Verification items for the finished model (mm, model axes). Face numbers are marked on the shaded views. Round coordinates to 2 decimals unless told otherwise and drop trailing zeros. Loops run counter-clockwise (first coordinate to the right, second up) from the corner with the lowest first, then second, coordinate; pieces in that order, holes last. Notation, with made-up numbers: M 19.25,9 L 50.25,9 A15 ccw 50.25,35 Z; hole C 2.25,23.25 d4. An arc over 180 degrees is marked long. One line per item, written item: value.
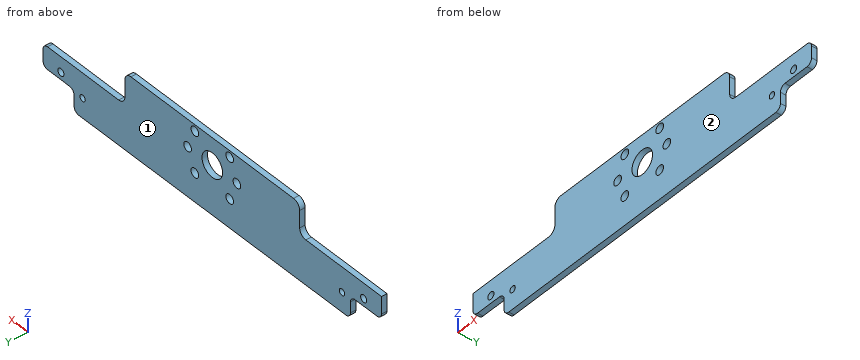
from build123d import *

# Parameters (mm, degrees)
SKETCH_2_R      = 2.5
SKETCH_2_R_2    = 2.499999999
SKETCH_2_R_3    = 6.682030953
SKETCH_2_R_4    = 2
SKETCH_2_R_5    = 1.75
EXTRUDE_1_DEPTH = 3
FILLET_1_R      = 4
FILLET_2_R      = 3


with BuildPart() as part:
    # 草图2 → 凸台-拉伸1 (new body)
    with BuildSketch(Plane(origin=(0, 0, 0), x_dir=(1, 0, 0), z_dir=(0, 1, 0))):
        Polygon((56.805521657, -9.129480985), (110, -9.129480985), (110, 3.251695679), (89.78, 3.370519015), (89.78, 15.370519015), (-89.78, 15.370519015), (-89.78, 3.370519015), (-110, 3.370519015), (-110, -9.129480985), (-56.805521657, -9.129480985), (-56.805521657, -26.629480985), (56.805521657, -26.629480985), align=None)
        with Locations((-16.000000001, -11.748304322)):
            Circle(SKETCH_2_R, mode=Mode.SUBTRACT)
        with Locations((-11.313708499, -23.062012821)):
            Circle(SKETCH_2_R_2, mode=Mode.SUBTRACT)
        with Locations((-11.3137085, -0.434595823)):
            Circle(SKETCH_2_R, mode=Mode.SUBTRACT)
        with Locations((0, -11.748304321)):
            Circle(SKETCH_2_R_3, mode=Mode.SUBTRACT)
        with Locations((11.313708498, -0.434595822)):
            Circle(SKETCH_2_R, mode=Mode.SUBTRACT)
        with Locations((16, -11.748304321)):
            Circle(SKETCH_2_R, mode=Mode.SUBTRACT)
        with Locations((11.313708499, -23.062012821)):
            Circle(SKETCH_2_R_2, mode=Mode.SUBTRACT)
        with Locations((98.383175919, -0.748304322)):
            Circle(SKETCH_2_R_4, mode=Mode.SUBTRACT)
        with Locations((84.28, 4.561107346)):
            Circle(SKETCH_2_R_5, mode=Mode.SUBTRACT)
        with Locations((-84.280000001, 4.561107346)):
            Circle(SKETCH_2_R_5, mode=Mode.SUBTRACT)
        with Locations((-98.38317592, -0.748304322)):
            Circle(SKETCH_2_R_4, mode=Mode.SUBTRACT)
    extrude(amount=EXTRUDE_1_DEPTH)

    # 圆角1
    fillet_1_edges = [part.edges().sort_by_distance(p)[0] for p in [
        (56.805521657, 1.5, 9.129480985),
        (56.805521657, 1.5, 26.629480985),
        (-56.805521657, 1.5, 26.629480985),
        (-56.805521657, 1.5, 9.129480985),
    ]]
    fillet(fillet_1_edges, radius=FILLET_1_R)

    # 圆角2
    fillet_2_edges = [part.edges().sort_by_distance(p)[0] for p in [
        (89.78, 1.5, -3.370519015),
        (110, 1.5, -3.251695679),
        (110, 1.5, 9.129480985),
        (-110, 1.5, -3.370519015),
        (-89.78, 1.5, -3.370519015),
        (-89.78, 1.5, -15.370519015),
        (89.78, 1.5, -15.370519015),
    ]]
    fillet(fillet_2_edges, radius=FILLET_2_R)


solid = part.part
(1) Sectioned sample at C-C on z = -8.5. Enter the section's corners in (x, y).
Completed:
outline: M -89.78,0 L 89.78,0 L 89.78,3 L -89.78,3 Z
(2) Sectioned sample at D-D on x = 68. Enter the section's corners in (y, z), and give its area (3 significant figures).
Completed:
outline: M 0,-15.37 L 3,-15.37 L 3,9.13 L 0,9.13 Z
area: 73.5 mm^2
(3) Thickness scan on L1, parallel to Z at x = 98.5, y = 0.6; L2, parallel to Z at x = 84.5, y = 1.8 (3 decimals); L3, parallel to X at y = 1.7, z = -6. Record the ranges inside material, lowest first. Write a range as from..to.
Completed:
L1: z = -3.32..-1.25, 2.74..9.13
L2: z = -15.371..-6.297, -2.825..9.129
L3: x = -89.8..-85.28, -83.28..83.28, 85.28..89.8
(4) Sectioned sample at B-B on y = 2.45. Count the separate pieces of the cut face and the enclosed holes in it, and give its area (3 significant figures).
Completed:
separate pieces: 1
enclosed holes: 11
area: 6,580 mm^2
(5) Mould release check, pull along Y, two halves, no side actions. Record for the marked faces 1 and 2: +Y half, -Y half, draft (parallel to the pull), parting line (faces both ways), or undercut.
Completed:
face 1: +Y half
face 2: -Y half
(6) Depth check by flat-ended pin: pin 1 Ø1.5 at (y, z) = (1, 16) entering from -X; pin 2 Ø1.5 at (y, z) = (2, -9) entering from +X; pin 3 Ø3 at (x, z) = (-98.38, 0.75) entering from -Y (3 decimals); pin 4 Ø1.5 at (y, z) = (1, 18) entering from +X. Enter the tip coordinate at first touch or a pass-through.
Completed:
pin 1: stops at x = -56.81
pin 2: stops at x = 89.78
pin 3: passes through
pin 4: stops at x = 56.81
(7) Sectioned sample at A-A on x = 0. Enter the section's corners in (y, z), and give its area (3 significant figures).
Completed:
outline: M 0,-15.37 L 3,-15.37 L 3,5.07 L 0,5.07 Z; M 0,18.43 L 3,18.43 L 3,26.63 L 0,26.63 Z
area: 85.9 mm^2
